from build123d import *

# Parameters (mm, degrees)
TROU_DE_PASSAGE_D_AXE_3_321_REACH  = 32.636
TROU_DE_PASSAGE_D_AXE_3_321_BORE_R = 5
TROU_DE_PASSAGE_D_AXE_3_322_D      = 14.5


with BuildPart() as part:
    # Esquisse1 → Révolution1 (revolve)
    with BuildSketch(Plane(origin=(0, 0, 0), x_dir=(1, 0, 0), z_dir=(0, 1, 0)), mode=Mode.PRIVATE) as r_volution1_sk:
        Polygon((7.250000000000006, 51.46955999467971), (7.2500000000000115, 16.46955999467971), (9.250000000000007, 16.46955999467971), (9.250000000000007, 51.46955999467971), align=None)
    revolve(r_volution1_sk.sketch.rotate(Axis((0, 0, -65.50671272050145), (0, 0, 1)), 180), axis=Axis((0, 0, -65.50671272050145), (0, 0, 1)))

    # Trou de passage d'axe 3/321 bore (on position points) → Trou de passage d'axe 3/321 (cut, up to next)
    with BuildSketch(Plane(origin=(-5.876504309, -7.143472342, -30.469559995), x_dir=(-0.772267280236, 0.635297763161, 0), z_dir=(-0.635297763161, -0.772267280236, 0)), mode=Mode.PRIVATE) as trou_de_passage_d_axe_3_321_sk1:
        Circle(TROU_DE_PASSAGE_D_AXE_3_321_BORE_R)
    trou_de_passage_d_axe_3_321_tool1 = extrude(trou_de_passage_d_axe_3_321_sk1.sketch, amount=-TROU_DE_PASSAGE_D_AXE_3_321_REACH, mode=Mode.PRIVATE) & part.part
    add(trou_de_passage_d_axe_3_321_tool1.solids().sort_by_distance((-5.876504, -7.143472, -30.46956))[0], mode=Mode.SUBTRACT)

    # Esquisse6 → Révolution2 (revolve)
    with BuildSketch(Plane(origin=(0, 0, 0), x_dir=(0, 0, -1), z_dir=(0.7722672802355546, -0.6352977631611647, 0)), mode=Mode.PRIVATE) as r_volution2_sk:
        Polygon((22.469559994679706, -16.22010142633931), (22.469559994679706, -17.826400392261572), (11.469559994679708, -17.826400392261572), (11.469559994679708, -22.802862204144958), (10.469559994679706, -22.802862204144958), (10.469559994679706, -16.826400392261576), (21.469559994679706, -16.826400392261572), (21.469559994679706, -16.22010142633931), (21.469559994679706, -3.2201014263393115), (22.469559994679706, -3.2201014263393115), align=None)
    revolve(r_volution2_sk.sketch.rotate(Axis((-13.132857470311126, -15.964287470260585, -30.469559994679706), (0.6352977631611647, 0.7722672802355546, 0)), 90), axis=Axis((-13.132857470311126, -15.964287470260585, -30.469559994679706), (0.6352977631611647, 0.7722672802355546, 0)))

    # Trou de passage d'axe 3/322 (through all)
    with Locations(Plane(origin=(0, 0, -39.469559995), x_dir=(0, -1, 0), z_dir=(0, 0, -1))):
        with Locations((0, 0)):
            Hole(TROU_DE_PASSAGE_D_AXE_3_322_D / 2)


solid = part.part
Here's how the part is built. I have some questions about the finished solid (model axes, mm). A direction names the side the tool comes from. Give positions to 0.01 mm unless a question says otherwise; leave off trailing zeros. Loops run counter-clockwise (first coordinate to the right, second up) from the corner with the lowest first, then second, coordinate; pieces in that order, holes last. Notation, with made-up numbers: (68, 26.25) -> (94, 26.25) arc R25 cw to (94, 48.25) -> close; hole circle Ø4 at (18.25, 31). An arc over 180 degrees is marked (long way). Answer as a JSON object with one key per item and string values. Group by question number.
Item 1: Imagine slicing it at C-C on z = -13. Write out the boundary of the cut face in (x, y).
Item 2: Imagine slicing it at D-D on y = -3.5. Give the number of separate pieces and of enclosed holes in the cut face, then the cut area to 3 significant figures.
Item 3: Imagine slicing it at B-B on y = 4. Write out the boundary of the cut face in (x, z), then the cut area to 3 significant figures.
Item 4: On a 3-axis mill with a long thin cutter (end or side, diameter ignored), from which of +Z, -Z, +X, -X, +Y, -Y can I reach the whole of each face in a straight line? I mean faces 1 (the flat face through (-4, -18.5, -26.3)), 2 (the flat face through (6, 5, -51.47)). Say none if no direction works.
Item 5: Will these pins go through, and if not, where does the flat tip stop? pin 1 (12 mm diameter, centred on x = -12.5, y = 0, fed in from +Z); pin 2 (2 mm diameter, centred on y = 2, z = -38.5, fed in from +X); pin 3 (1.5 mm diameter, centred on x = -26, z = -27.5, fed in from -Y); pin 4 (8.5 mm diameter, centred on x = 0, y = 0, fed in from +Z).
Item 6: Imagine slicing it at A-A on z = -41. Write out the boundary of the cut face in (x, y), then the cut area to 3 significant figures.
Item 7: Thinking about a two-plate mould opening in Y: for faces 3 (the cylindrical face through (-5.435, -21.133, -12.726)), 4 (the flat face through (-22.423, -11.081, -14.267)), 5 (the cylindrical face through (-3.09, 6.56, -33.72)), 6 (the flat face through (-6, 5, -16.47)), which applies, pulls with the +Y half, pulls with the -Y half, needs draft (parallel to the pull), parting line crosses it, or undercut?
Item 8: I need wall thicknesses on L1, parallel to Y at x = 0, z = -22.5; L2, parallel to Y at x = 0, z = -34.5; L3, parallel to Y at x = 0, z = -43. Which ranges of each line are inside material? Lowest first, please.
Answer list:
{
 "1": {"outline": "(-22.01, -11.42) -> (-20.26, -12.86) -> (-17.09, -9.02) -> (-5.56, -18.51) -> (-8.72, -22.36) -> (-6.97, -23.8) -> (-3.17, -19.18) -> (-18.21, -6.81) -> close"},
 "2": {"separate pieces": "3", "enclosed holes": "1", "area": "232 mm2"},
 "3": {"outline": "(-8.34, -51.47) -> (-6.05, -51.47) -> (-6.05, -16.47) -> (-8.34, -16.47) -> close; (6.05, -51.47) -> (8.34, -51.47) -> (8.34, -16.47) -> (6.05, -16.47) -> close", "area": "161 mm2"},
 "4": {"face 1": "none", "face 2": "-Z, +X, -X, +Y, -Y"},
 "5": {"pin 1": "stops at z = -16.47", "pin 2": "stops at x = 9.2", "pin 3": "stops at y = -3", "pin 4": "passes through"},
 "6": {"outline": "(-27.62, -6.81) -> (-26.7, -7.56) -> (-23.54, -3.72) -> (0.89, -23.81) -> (-2.27, -27.66) -> (-1.36, -28.41) -> (2.44, -23.8) -> (-23.82, -2.19) -> close; circle Ø18.5 at (0, 0); hole circle Ø14.5 at (0, 0)", "area": "150 mm2"},
 "7": {"face 3": "parting line crosses it", "face 4": "pulls with the -Y half", "face 5": "undercut", "face 6": "needs draft"},
 "8": {"L1": "y = -28.87 to -27.15, -23.08 to -21.79, -9.25 to -7.25, 7.25 to 9.25", "L2": "y = -29.53 to -29.23, -23.08 to -21.79, -12.67 to -10.88, -9.25 to -7.25, 7.25 to 9.25", "L3": "y = -24.54 to -21.79, -9.25 to -7.25, 7.25 to 9.25"}
}
